Verification items for the finished model (mm, model axes). Face numbers are marked on the shaded views. A direction names the side the tool comes from. Give positions to 0.01 mm unless a question says otherwise; leave off trailing zeros. Write each loop counter-clockwise with the first axis right and the second up, starting at its lowest first coordinate (ties: lowest second). Pieces come first, ordered by that corner, then holes. Notation, with made-up numbers: (-8.75, 63.25) -> (43.25, 63.25) arc R10 cw to (43.25, 74.25) -> close; hole circle Ø11 at (65, 72). An arc over 180 degrees is marked (long way). Answer as CSV lines item,"result".
```python
from build123d import *

# Parameters (mm, degrees)
BOSS_EXTRUDE1_DEPTH     = 18
SKETCH2_R               = 5.25
CUT_EXTRUDE1_DEPTH      = 52.54422425
CUT_EXTRUDE2_START      = -10
CUT_EXTRUDE2_DEPTH      = 10
CUT_EXTRUDE3_DEPTH      = 52.54422425
CUT_EXTRUDE4_DEPTH      = 52.544224284
SKETCH6_R               = 3
CUT_EXTRUDE5_DEPTH      = 10
CUT_EXTRUDE6_REACH      = 52.806
CUT_EXTRUDE6_END_RADIUS = 19
SKETCH7_R               = 1.5


# Read off the part's stored shape, not the designer's step: Cut-Extrude2
with BuildPart() as part:
    # Sketch1 → Boss-Extrude1 (new, symmetric)
    with BuildSketch(Plane.XY):
        with BuildLine():
            Line((22.627416998, 17.790398646), (42.997756377, 17.790398646))
            Line((42.997756377, 17.790398646), (42.997756377, 7.790398646))
            Line((42.997756377, 7.790398646), (21.997756377, 7.790398646))
            Line((21.997756377, 7.790398646), (21.997756377, -4.209601354))
            Line((21.997756377, -4.209601354), (18.027756377, -4.209601354))
            ThreePointArc((18.027756377, -4.209601354), (0, 8.790398646), (-18.027756377, -4.209601354))
            Line((-18.027756377, -4.209601354), (-21.997756377, -4.209601354))
            Line((-21.997756377, -4.209601354), (-21.997756377, 7.790398646))
            Line((-21.997756377, 7.790398646), (-42.997756377, 7.790398646))
            Line((-42.997756377, 7.790398646), (-42.997756377, 17.790398646))
            Line((-42.997756377, 17.790398646), (-22.627416998, 17.790398646))
            ThreePointArc((-22.627416998, 17.790398646), (0, 25.790398646), (22.627416998, 17.790398646))
        make_face()
    extrude(amount=BOSS_EXTRUDE1_DEPTH, both=True)

    # Sketch2 → Cut-Extrude1 (cut, through all)
    with BuildSketch(Plane(origin=(0, 17.790398646, 0), x_dir=(1, 0, 0), z_dir=(0, 1, 0))):
        with Locations(Location((-31, 0, 0), (0, 0, 180))):
            Circle(SKETCH2_R)
        with Locations(Location((31, 0, 0), (0, 0, 180))):
            Circle(SKETCH2_R)
    extrude(amount=-CUT_EXTRUDE1_DEPTH, mode=Mode.SUBTRACT)

    # Cut-Extrude2 outline → Cut-Extrude2 (cut)
    with BuildSketch(Plane(origin=(0, 17.790398646, 0), x_dir=(1, 0, 0), z_dir=(0, 1, 0)).offset(CUT_EXTRUDE2_START)):
        with BuildLine():
            ThreePointArc((39.05124838, 18), (41.953602003, 9.428429295), (42.997756377, 0.439256778))
            Line((42.997756377, 0.439256778), (42.997756377, 18))
            Line((42.997756377, 18), (39.05124838, 18))
        make_face()
        with BuildLine():
            Line((42.997756377, -18), (42.997756377, -0.439256778))
            ThreePointArc((42.997756377, -0.439256778), (41.953602003, -9.428429295), (39.05124838, -18))
            Line((39.05124838, -18), (42.997756377, -18))
        make_face()
        with BuildLine():
            ThreePointArc((-42.997756377, 0.439256778), (-41.953602003, 9.428429295), (-39.05124838, 18))
            Line((-39.05124838, 18), (-42.997756377, 18))
            Line((-42.997756377, 18), (-42.997756377, 0.439256778))
        make_face()
        with BuildLine():
            Line((-42.997756377, -18), (-39.05124838, -18))
            ThreePointArc((-39.05124838, -18), (-41.953602003, -9.428429295), (-42.997756377, -0.439256778))
            Line((-42.997756377, -0.439256778), (-42.997756377, -18))
        make_face()
    extrude(amount=CUT_EXTRUDE2_DEPTH, mode=Mode.SUBTRACT)

    # Sketch4 → Cut-Extrude3 (cut, through all)
    with BuildSketch(Plane(origin=(0, 17.790398646, 0), x_dir=(1, 0, 0), z_dir=(0, 1, 0))):
        with BuildLine():
            Line((-22.627416998, 8.596502421), (-22.627416998, -8.596502421))
            ThreePointArc((-22.627416998, -8.596502421), (-19, 0), (-22.627416998, 8.596502421))
        make_face()
    extrude(amount=CUT_EXTRUDE3_DEPTH, mode=Mode.SUBTRACT)

    # Sketch5 → Cut-Extrude4 (cut, through all)
    with BuildSketch(Plane(origin=(0, 17.790398646, 0), x_dir=(1, 0, 0), z_dir=(0, 1, 0))):
        with BuildLine():
            Line((22.627416998, 8.596502421), (22.627416998, -8.596502421))
            ThreePointArc((22.627416998, -8.596502421), (19, 0), (22.627416998, 8.596502421))
        make_face()
    extrude(amount=CUT_EXTRUDE4_DEPTH, mode=Mode.SUBTRACT)

    # Sketch6 → Cut-Extrude5 (cut)
    with BuildSketch(Plane(origin=(0, 26, 0), x_dir=(1, 0, 0), z_dir=(0, 1, 0))):
        with Locations(Location((0, 0, 0), (0, 0, 270))):
            Circle(SKETCH6_R)
    extrude(amount=-CUT_EXTRUDE5_DEPTH, mode=Mode.SUBTRACT)

    # Cut-Extrude6: up to this cylinder (the profile starts outside it)
    cut_extrude6_end = Plane(origin=(0, -10.209601354, 0), z_dir=(0, 0, -1)) * Cylinder(CUT_EXTRUDE6_END_RADIUS, 144.612, mode=Mode.PRIVATE)
    # Sketch7 → Cut-Extrude6 (cut, up to the surface)
    with BuildSketch(Plane(origin=(0, 16, 0), x_dir=(1, 0, 0), z_dir=(0, 1, 0)), mode=Mode.PRIVATE) as cut_extrude6_sk1:
        with Locations(Location((0, 0, 0), (0, 0, 270))):
            Circle(SKETCH7_R)
    cut_extrude6_tool1 = extrude(cut_extrude6_sk1.sketch, amount=-CUT_EXTRUDE6_REACH, mode=Mode.PRIVATE) - cut_extrude6_end
    add(cut_extrude6_tool1.solids().sort_by_distance((0, 16, 0))[0], mode=Mode.SUBTRACT)


solid = part.part
```
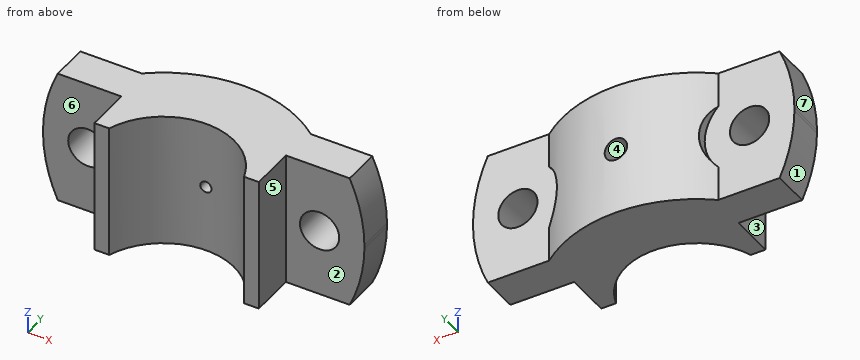
1) Section check B-B (y = 2.5). Record the boundary of the cut face in (x, z), and give its area (3 significant figures).
Reported:
outline,"(-22, -18) -> (-14.12, -18) -> (-14.12, 18) -> (-22, 18) -> close; (14.12, -18) -> (22, -18) -> (22, 18) -> (14.12, 18) -> close"
area,"567 mm²"
2) Scan lines: line 1 along Z through (x, y) = (31, 14); line 2 along Z through (x, y) = (0, 18); line 3 along Y through (x, z) = (-35, 6). Record each from-to range of solid material in increasing order.
Reported:
line 1,"-18 to -5.25, 5.25 to 18"
line 2,"-18 to -3, 3 to 18"
line 3,"7.79 to 17.79"
3) Draft check along X on the marked faces 4, 5, 6 and 7. Enter one of: +X half, -X half, draft (parallel to the pull), parting line (faces both ways), or undercut.
Reported:
face 4,"undercut"
face 5,"+X half"
face 6,"draft"
face 7,"-X half"
4) Section check D-D (x = 0). Record the boundary of the cut face in (y, z).
Reported:
outline,"(8.79, -18) -> (25.79, -18) -> (25.79, -3) -> (16, -3) -> (16, -1.5) -> (8.79, -1.5) -> close; (8.79, 1.5) -> (16, 1.5) -> (16, 3) -> (25.79, 3) -> (25.79, 18) -> (8.79, 18) -> close"
5) Section check C-C (z = 4). Record the boundary of the cut face in (x, y).
Reported:
outline,"(-42.81, 7.79) -> (-34.4, 7.79) -> (-34.4, 17.79) -> (-42.81, 17.79) -> close; (-27.6, 7.79) -> (-22, 7.79) -> (-22, -4.21) -> (-18.03, -4.21) arc R19 cw to (18.03, -4.21) -> (22, -4.21) -> (22, 7.79) -> (27.6, 7.79) -> (27.6, 17.79) -> (19.69, 17.79) -> (19.69, 19.93) arc R36 ccw to (-19.69, 19.93) -> (-19.69, 17.79) -> (-27.6, 17.79) -> close; (34.4, 7.79) -> (42.81, 7.79) -> (42.81, 17.79) -> (34.4, 17.79) -> close"
6) Section check A-A (x = 31). Record the boundary of the cut face in (y, z), and give its area (3 significant figures).
Reported:
outline,"(7.79, -18) -> (17.79, -18) -> (17.79, -5.25) -> (7.79, -5.25) -> close; (7.79, 5.25) -> (17.79, 5.25) -> (17.79, 18) -> (7.79, 18) -> close"
area,"255 mm²"
7) Tool access check on the marked faces 1, 2 and 3. Record the directions out of +Z, -Z, +X, -X, +Y, -Y that give a thin tool (end or side, any length) a straight path to the whole face; none if there is none.
Reported:
face 1,"-Z, -X, +Y, -Y"
face 2,"+Z, -Z, +X, -Y"
face 3,"+Z, -Z, -X, -Y"
8) Depth check by flat-ended pin: pin 1 (8 mm diameter, centred on x = -33.5, z = 5, fed in from +Y); pin 2 (2.5 mm diameter, centred on x = 0, z = 0, fed in from -Y); pin 3 (10.5 mm diameter, centred on x = -28, z = 2.5, fed in from -Y); pin 4 (3 mm diameter, centred on y = 13, z = 9.5, fed in from +X). Enter the tip coordinate at first touch or a pass-through.
Reported:
pin 1,"y = 17.79"
pin 2,"through"
pin 3,"y = 7.79"
pin 4,"x = 42.25"
